Source: three-view drawing plus pictorial views. Frame: mm from the lowest corner of the part. A direction names the side the tool comes from. Give positions to 0.01 mm unless a question says otherwise; leave off trailing zeros. Loops run counter-clockwise (first coordinate to the right, second up) from the corner with the lowest first, then second, coordinate; pieces in that order, holes last.
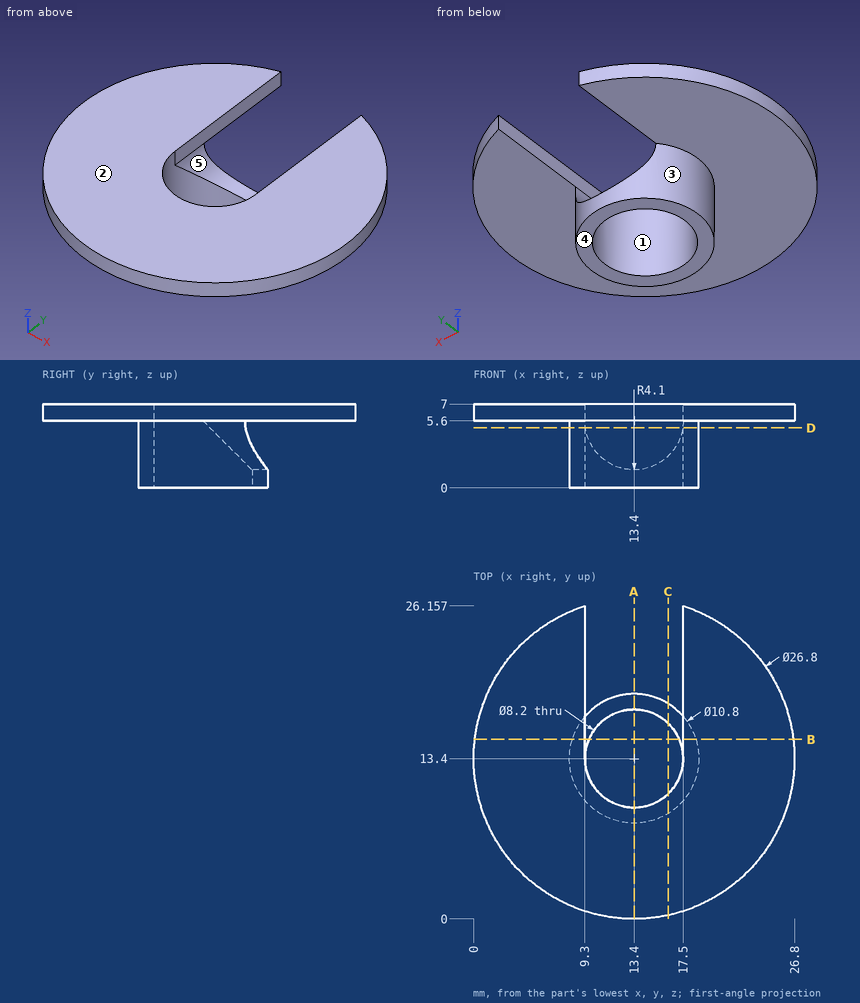
(1) Ray query, probe 1 along X at (y, z) = (13.4, 4.75); probe 2 along Y at (x, z) = (13.4, 1.75); probe 3 along Z at (x, y) = (4.75, 23.5). Return the intervals inside material, ascending.
Values follow:
probe 1: x = 8 to 9.3, 17.5 to 18.8
probe 2: y = 8 to 9.3
probe 3: z = 5.6 to 7
(2) Cut plane B-B (y = 15). Return the cut outline in (x, z) (1 decimal).
Values follow:
outline: (0.1, 5.6) - (8.2, 5.6) - (8.2, 0) - (9.6, 0) - (9.6, 4) arc R4.1 cw to (9.3, 5.6) - (9.3, 7) - (0.1, 7) - close; (17.2, 0) - (18.6, 0) - (18.6, 5.6) - (26.7, 5.6) - (26.7, 7) - (17.5, 7) - (17.5, 5.6) arc R4.1 cw to (17.2, 4) - close
(3) Cut plane C-C (x = 16.25). Return the cut outline in (y, z).
Values follow:
outline: (0.31, 5.6) - (8.81, 5.6) - (8.81, 0) - (10.45, 0) - (10.45, 7) - (0.31, 7) - close; (16.35, 0) - (17.99, 0) - (17.99, 2.65) - (16.35, 2.65) - close
(4) Mould query, pull axis Y, two halves, no side actions, for the marked faces 1, 2 and 3. Classes: +Y half, -Y half, draft (parallel to the pull), parting line (faces both ways), or undercut.
Values follow:
face 1: undercut
face 2: draft
face 3: parting line
(5) Cut plane D-D (z = 5). Return the cut outline in (x, y) (1 decimal).
Values follow:
outline: (9.3, 14) - (9.3, 17) arc R5.4 ccw (long way) to (17.5, 17) - (17.5, 14) arc R4.1 cw (long way) to start
(6) Pin query (flat end, axial travel): pin 1 Ø1.5 at (y, z) = (18, 6.5) entering from +X (1 decimal); pin 2 Ø3 at (y, z) = (11, 3) entering from -X (1 decimal); pin 3 Ø2 at (x, z) = (7.5, 3) entering from -Y; pin 4 Ø1.5 at (x, z) = (6.5, 1) entering from -Y. Return the tip coordinate at first contact, or that it passes through.
Values follow:
pin 1: stops at x = 26.2
pin 2: stops at x = 8.1
pin 3: stops at y = 11.13
pin 4: passes through
(7) Reachability of the marked faces 4 and 5 from +Z, -Z, +X, -X, +Y, -Y: full face, straight path, thin tool, end or side. Return the list, or none.
Values follow:
face 4: -Z, +X, -X, +Y, -Y
face 5: +Z, +Y
(8) Cut plane A-A (x = 13.4). Return the cut outline in (y, z).
Values follow:
outline: (0, 5.6) - (8, 5.6) - (8, 0) - (9.3, 0) - (9.3, 7) - (0, 7) - close; (17.5, 0) - (18.8, 0) - (18.8, 1.5) - (17.5, 1.5) - close
